Input: part model. Units: mm. Frame: model coordinates. A direction names the side the tool comes from. Round coordinates to 2 decimals unless told otherwise and drop trailing zeros. Write each loop counter-clockwise with the first axis right and the second up, starting at its lowest first coordinate (ties: lowest second). Pieces come first, ordered by that corner, then holes. Notation, with made-up numbers: M -34,86 L -17,86 A17 ccw -17,99 Z; hole C -6,63.5 d5. An arc over 180 degrees is marked long. Write each question's results on one line, items separated by ' | '. Start each with the question number.
Autodesk Fusion 360 part; units mm, degrees
sketch "Sketch1" plane through (0, 0, 0) normal (0, 0, 1) x (1, 0, 0)
  line L0 (0, 0) -> (50, 0)
  line L1 (0, 0) -> (-50, 0)
  line L2 (0, -60) -> (50, -60)
  line L3 (0, -60) -> (-50, -60)
  line L4 (0, -2.5) -> (47.5, -2.5)
  line L5 (0, -2.5) -> (-47.5, -2.5)
  line L6 (0, -57.5) -> (47.5, -57.5)
  line L7 (0, -57.5) -> (-47.5, -57.5)
  line L8 (-47.5, -2.5) -> (-47.5, -57.5)
  line L9 (47.5, -2.5) -> (47.5, -57.5)
  line L10 (50, -60) -> (50, 0)
  line L11 (-50, -60) -> (-50, 0)
  line L12 (-54.3467, -2.5) -> (-57.3288, -2.5) construction
  line L13 (-47.5, -22.5) -> (47.5, -22.5)
  line L14 (-47.5, 10.1561) -> (-47.5, 7.5248)
  line L15 (-47.5, -22.5) -> (-27.5, -2.5)
  line L16 (27.5, -2.5) -> (27.5, -7.3859)
  line L17 (47.5, -22.5) -> (27.5, -2.5)
  line L18 (-47.5, -37.5) -> (-27.9827, -57.5)
  line L19 (47.5, -37.5) -> (-47.5, -37.5)
  line L20 (27.5, -57.5) -> (47.5, -37.5)
  dimension "d1" = 50
  dimension "d2" = 50
  dimension "d3" = 60
  dimension "d4" = 50
  dimension "d5" = 50
  dimension "d6" = 2.5
  dimension "d7" = 47.5
  dimension "d8" = 47.5
  dimension "d9" = 2.5
  dimension "d10" = 47.5
  dimension "d11" = 47.5
extrude "Extrude1" add sketch "Sketch1" along normal blind 10
extrude "Extrude2" add sketch "Sketch1" along normal blind 25 contours L4 L9 L17 | L5 L8 L15 | L6 L9 L20 | L7 L8 L18
extrude "Extrude3" add sketch "Sketch1" along normal blind 2.5 contours L4 L5 L13 L15 L17 | L8 L9 L13 L19 | L6 L7 L18 L19 L20
1. Cut plane D-D on y = -29.5. Output: boundary loops of the cut face in (x, z), and give its area (4 significant figures).
2. Access query for faces 4 (the face through (-47.5, -47, 17)), 5 (the face through (47.5, -47, 17)), 6 (the face through (-1, -30, 2.5)), 7 (the face through (-38, -57.5, 17)), 8 (the face through (37, -2.5, 17)). Directions: +Z, -Z, +X, -X, +Y, -Y. A direction counts if a zero-diameter tool reaches every point of the face in a straight line with its end or side. Return the directions, or none.
3. Draft query along X for faces 1 (the face through (-1, -30, 0)), 2 (the face through (50, -30, 5)), 3 (the face through (-37.88, -47.36, 13.59)). Return one class per face: +X half, -X half, draft (parallel to the pull), parting line (faces both ways), or undercut.
4. Cut plane C-C on z = 23.75. Output: boundary loops of the cut face in (x, y).
5. Contact query for flat-ended pins moving along their axis: P1, Ø3, axis at x = -35, y = -15, coming from the +Z side; P2, Ø7.5, axis at y = -9, z = 14, coming from the -X side; P3, Ø10, axis at x = -32, z = 21, coming from the +Y side. Output: stop coordinate, or through.
6. Cut plane A-A on x = -15. Output: boundary loops of the cut face in (y, z), and give its area (4 significant figures).
7. Cut plane B-B on z = 7. Output: boundary loops of the cut face in (x, y).
8. Line query: L1, parallel to Y at x = 9, z = 4; L2, parallel to X at y = -29, z = 8; L3, parallel to Z at x = -41.5, y = -18. Output: solid intervals per line, ascending. Write a range as from..to.
Answers follow:
1) outline: M -50,0 L 50,0 L 50,10 L 47.5,10 L 47.5,2.5 L -47.5,2.5 L -47.5,10 L -50,10 Z | area: 287.5 mm2
2) face 4: +Z, -X, +Y, -Y | face 5: +Z, +X, +Y, -Y | face 6: +Z | face 7: +Z, +X, -X, -Y | face 8: +Z, +X, -X, +Y
3) face 1: draft | face 2: +X half | face 3: undercut
4) outline: M -47.5,-57.5 L -27.98,-57.5 L -47.5,-37.5 Z; M -47.5,-22.5 L -27.5,-2.5 L -47.5,-2.5 Z; M 27.5,-57.5 L 47.5,-57.5 L 47.5,-37.5 Z; M 27.5,-2.5 L 47.5,-22.5 L 47.5,-2.5 Z
5) P1: stops at z = 2.5 | P2: stops at x = -47.5 | P3: stops at y = -2.5
6) outline: M -60,0 L 0,0 L 0,10 L -2.5,10 L -2.5,2.5 L -57.5,2.5 L -57.5,10 L -60,10 Z | area: 187.5 mm2
7) outline: M -50,-60 L 50,-60 L 50,0 L -50,0 Z; hole M -47.5,-37.5 L -27.98,-57.5 L 27.5,-57.5 L 47.5,-37.5 L 47.5,-22.5 L 27.5,-2.5 L -27.5,-2.5 L -47.5,-22.5 Z
8) L1: y = -60..-57.5, -2.5..0 | L2: x = -50..-47.5, 47.5..50 | L3: z = 0..2.5
